Build history of the part. All positions in model axes, mm. A direction names the side the tool comes from. Coordinates: 2 decimals unless noted, no trailing zeros. Order: outer loops, then holes, each group sorted by start corner. A loop starts at its lowest first (then second) coordinate and runs counter-clockwise, first axis right, second up. Notation, with made-up numbers: (63.25, 15) -> (72.25, 15) arc R24 ccw to (72.25, 47) -> close; hole circle Ø2 at (58, 61). An arc over 180 degrees is marked (long way). Write each question's results on one line, items separated by ' | '.
from build123d import *

# Parameters (mm, degrees)
F4_DEPTH = 2
F5_DEPTH = 2
F6_COUNT = 2
F6_ANGLE = 60
F8_DEPTH = 2
F9_COUNT = 3
F9_ANGLE = 240


with BuildPart() as f4:
    # F3 (on Top) → F4 (new body)
    with BuildSketch(Plane.XY):
        Polygon((-8, 4.6188021535), (-20, 11.5470053838), (-20, -11.5470053838), (-8, -4.6188021535), align=None)
        Polygon((-18, -9.237604307), (-18, 9.237604307), (-10, 4.6188021535), (-10, -4.6188021535), align=None, mode=Mode.SUBTRACT)
        Polygon((-10, 4.6188021535), (-18, 9.237604307), (-18, -9.237604307), (-10, -4.6188021535), align=None)
    extrude(amount=F4_DEPTH)

    # F3 (on Top) → F5 (join)
    with BuildSketch(Plane.XY):
        Polygon((-20, -11.5470053838), (-20, 11.5470053838), (-22, 12.7017059222), (-22, -12.7017059222), align=None)
    extrude(amount=F5_DEPTH)

    # F6: F4 ×2 about axis
    f6_axis = Axis((0, 0, 0), (0, 0, 1))


with BuildPart() as f4_1:
    add(f4.part)
    for i in range(1, F6_COUNT):
        add(f4.part.rotate(f6_axis, i * F6_ANGLE / (F6_COUNT - 1)))

    # F7 (on Top) → F8 (join, through all)
    with BuildSketch(Plane.XY):
        Polygon((-24, 1.5588457268), (-22, 2.7135462652), (-22, 5.0229473419), (-24, 6.1776478803), (-24, 5.0229473419), (-24, 2.7135462652), align=None)
        Polygon((-24, -6.1776478803), (-22, -5.0229473419), (-22, -2.7135462652), (-24, -1.5588457268), (-24, -2.7135462652), (-24, -5.0229473419), align=None)
        Polygon((-19.7, -16.3390126181), (-17.7, -17.4937131564), (-16.7, -18.0710634256), (-16.7, -15.7616623489), (-18.7, -14.6069618105), (-20.7, -15.7616623489), align=None)
        Polygon((-13, -20.2072594216), (-11, -21.36195996), (-10, -21.9393102292), (-10, -19.6299091524), (-12, -18.4752086141), (-14, -19.6299091524), align=None)
        Polygon((-7.3, -23.498155956), (-6.3, -24.0755062252), (-4.3, -25.2302067636), (-3.3, -25.8075570328), (-3.3, -23.498155956), (-5.3, -22.3434554176), align=None)
    extrude(amount=F8_DEPTH)

    # F9: F4 ×3 about axis
    f9_axis = Axis((0, 0, 0), (0, 0, 1))


with BuildPart() as f4_2:
    add(f4_1.part)
    for i in range(1, F9_COUNT):
        add(f4_1.part.rotate(f9_axis, i * F9_ANGLE / (F9_COUNT - 1)))


solid = f4_2.part
Item 1: Slice it at A-A, the plane x = 9.5. List the corners of the cut face in (y, z).
Answer:
outline: (-22.23, 0) -> (-20.9, 0) -> (-20.9, 2) -> (-22.23, 2) -> close; (-19.92, 0) -> (19.92, 0) -> (19.92, 2) -> (-19.92, 2) -> close; (20.9, 0) -> (22.23, 0) -> (22.23, 2) -> (20.9, 2) -> close
Item 2: Pull direction X, two halves, no side cores. Call faces 1 (the flat face through (22.986, -9.46, 0.986)), 2 (the flat face through (-20.373, -13.641, 0.986)), 3 (the flat face through (-7.68, -20.97, 0.99)), 4 (the flat face through (-5, 10, 2)): released by +X, released by -X, zero draft, split by the parting line, or undercut.
Answer:
face 1: undercut | face 2: released by -X | face 3: undercut | face 4: zero draft
Item 3: Pin check, flat tips, straight feed: pin 1 (1 mm diameter, centred on y = -19, z = 1, fed in from -X) (3 decimals); pin 2 (0.6 mm diameter, centred on y = 11.5, z = 1.5, fed in from +X); pin 3 (0.6 mm diameter, centred on y = -1, z = 0.5, fed in from -X). Stop position of each tip, or through.
Answer:
pin 1: stops at x = -13.775 | pin 2: stops at x = 22 | pin 3: stops at x = -22
Item 4: Slice it at B-B, the plane y = 12. List the corners of the cut face in (x, z), and give its area (3 significant figures).
Answer:
outline: (-22, 0) -> (22, 0) -> (22, 2) -> (-22, 2) -> close | area: 88.0 mm^2
Item 5: Slice it at C-C, the plane x = -13. List the corners of the cut face in (y, z), and give its area (3 significant figures).
Answer:
outline: (-20.21, 0) -> (-19.05, 0) -> (-19.05, 2) -> (-20.21, 2) -> close; (-17.9, 0) -> (17.9, 0) -> (17.9, 2) -> (-17.9, 2) -> close; (19.05, 0) -> (20.21, 0) -> (20.21, 2) -> (19.05, 2) -> close | area: 76.2 mm^2
Item 6: Slice it at D-D, the plane x = 20. List the corners of the cut face in (y, z).
Answer:
outline: (-13.86, 0) -> (13.86, 0) -> (13.86, 2) -> (-13.86, 2) -> close
Item 7: Tool access for faces 5 (the flat face through (-5, 10, 0)), 6 (the flat face through (-20.327, 13.668, 0.986)): list every direction of +Z, -Z, +X, -X, +Y, -Y with a clear straight run to the whole face (end or side of a thin tool).
Answer:
face 5: -Z, +X, -X, +Y, -Y | face 6: +Z, -Z, -X
Item 8: Drill centre lines: line 1 (X direction, y = -3, z = 0.75); line 2 (X direction, y = -9, z = 1.25); line 3 (X direction, y = -6, z = 1.6). Where is each one in solid material? Low to high. Write a range as from..to.
Answer:
line 1: x = -24..-8, 8..22 | line 2: x = -22..-0.41, 0.41..22, 22.19..24 | line 3: x = -24..-23.69, -22..-5.61, 5.61..22, 23.01..24
